Check sheet for the modelled part. Datum: model origin and axes. Units: mm. Face numbers are marked on the shaded views. A direction names the side the tool comes from. Give positions to 0.01 mm unless a question says otherwise; leave off trailing zeros. Order: outer loops, then holes, each group sorted by start corner. A loop starts at its lowest first (then second) coordinate and runs counter-clockwise, first axis right, second up.
from build123d import *

# Parameters (mm, degrees)
BOSS_EXTRUDE1_DEPTH = 5
SKETCH2_W           = 0.4
SKETCH2_H           = 5
CUT_EXTRUDE1_DEPTH  = 3
SKETCH3_W           = 0.1
SKETCH3_H           = 5
CUT_EXTRUDE2_DEPTH  = 3
FILLET1_R           = 5
FILLET2_R           = 3


with BuildPart() as part:
    # Sketch1 → Boss-Extrude1 (new body)
    with BuildSketch(Plane.XY):
        Polygon((0, 65), (-28, 65), (-28, 57), (-8, 57), (-8, 8), (-28, 8), (-28, 0), (0, 0), (0, 57), (20, 57), (20, 65), align=None)
    extrude(amount=BOSS_EXTRUDE1_DEPTH)

    # Sketch2 → Cut-Extrude1 (cut)
    with BuildSketch(Plane(origin=(0, 8, 0), x_dir=(1, 0, 0), z_dir=(0, 1, 0))):
        with Locations((-23.8, -2.5)):
            Rectangle(SKETCH2_W, SKETCH2_H)
    extrude(amount=-CUT_EXTRUDE1_DEPTH, mode=Mode.SUBTRACT)

    # Sketch3 → Cut-Extrude2 (cut)
    with BuildSketch(Plane.XZ.offset(-57)):
        with Locations((-23.6, 2.5)):
            Rectangle(SKETCH3_W, SKETCH3_H)
    extrude(amount=-CUT_EXTRUDE2_DEPTH, mode=Mode.SUBTRACT)

    # Fillet1
    fillet1_edges = [part.edges().sort_by_distance(p)[0] for p in [
        (0, 0, 2.5),
        (-8, 8, 2.5),
        (-8, 57, 2.5),
        (0, 57, 2.5),
    ]]
    fillet(fillet1_edges, radius=FILLET1_R)

    # Fillet2
    fillet2_edges = [part.edges().sort_by_distance(p)[0] for p in [
        (-28, 57, 2.5),
        (-28, 65, 2.5),
        (20, 65, 2.5),
        (20, 57, 2.5),
    ]]
    fillet(fillet2_edges, radius=FILLET2_R)


solid = part.part
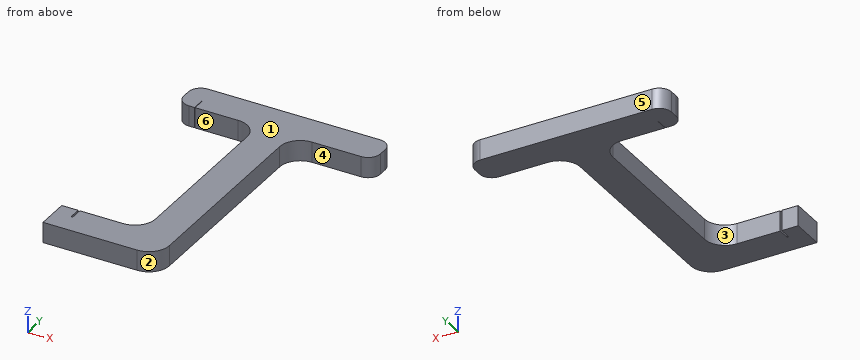
1) Material ranges on L1, parallel to Y at x = -25, z = 1.4; L2, parallel to Y at x = 8.5, z = 4.7; L3, parallel to X at y = 37.5, z = 0.65, recorded low to high.
Recorded:
L1: y = 0 to 8, 57 to 65
L2: y = 57 to 65
L3: x = -8 to 0
2) Set-up check for the marked faces 4, 5 and 6: record each of +Z, -Z, +X, -X, +Y, -Y from which the full face is reachable in a straight line by a thin tool's end or side.
Recorded:
face 4: +Z, -Z, +X, -Y
face 5: +Z, -Z, +X, -X, +Y
face 6: +Z, -Z, -X
3) Section check D-D, the plane x = 12. Record the cut outline in (y, z), then the cut area to 3 significant figures.
Recorded:
outline: (57, 0) - (65, 0) - (65, 5) - (57, 5) - close
area: 40.0 mm2
4) Section check A-A, the plane x = -19.5. Record the cut outline in (y, z).
Recorded:
outline: (0, 0) - (8, 0) - (8, 5) - (0, 5) - close; (57, 0) - (65, 0) - (65, 5) - (57, 5) - close
5) Section check C-C, the plane z = 2.35. Record the cut outline in (x, y).
Recorded:
outline: (-28, 0) - (-5, 0) arc R5 ccw to (0, 5) - (0, 52) arc R5 cw to (5, 57) - (17, 57) arc R3 ccw to (20, 60) - (20, 62) arc R3 ccw to (17, 65) - (-25, 65) arc R3 ccw to (-28, 62) - (-28, 60) arc R3 ccw to (-25, 57) - (-23.65, 57) - (-23.65, 60) - (-23.55, 60) - (-23.55, 57) - (-13, 57) arc R5 cw to (-8, 52) - (-8, 13) arc R5 cw to (-13, 8) - (-23.6, 8) - (-23.6, 5) - (-24, 5) - (-24, 8) - (-28, 8) - close
6) Draft check along Y on the marked faces 1, 2 and 3. Enter one of: +Y half, -Y half, draft (parallel to the pull), parting line (faces both ways), or undercut.
Recorded:
face 1: draft
face 2: -Y half
face 3: undercut
7) Section check B-B, the plane y = 7. Record the cut outline in (x, z), then the cut area to 3 significant figures.
Recorded:
outline: (-28, 0) - (-24, 0) - (-24, 5) - (-28, 5) - close; (-23.6, 0) - (0, 0) - (0, 5) - (-23.6, 5) - close
area: 138 mm2
8) Depth check by flat-ended pin: pin 1 Ø1.5 at (y, z) = (51.5, 1) entering from +X; pin 2 Ø6 at (x, y) = (13.5, 51.5) entering from +Z; pin 3 Ø2.5 at (x, z) = (10.5, 3.5) entering from -Y; pin 4 Ø2.5 at (y, z) = (58, 1.5) entering from +X. Enter the tip coordinate at first touch or a pass-through.
Recorded:
pin 1: stops at x = 0.01
pin 2: passes through
pin 3: stops at y = 57
pin 4: stops at x = 19.9
